Design review of the part built by this model. Coordinates are the model's own, in mm. A direction names the side the tool comes from. Round coordinates to 2 decimals unless told otherwise and drop trailing zeros. Order: outer loops, then holes, each group sorted by start corner. A loop starts at its lowest first (then second) coordinate and runs counter-clockwise, first axis right, second up. Notation, with made-up numbers: M 9.25,44 L 28.25,44 A15 cw 28.25,66 Z; hole C 43.25,7 d11. An arc over 180 degrees is marked long. Write each question's results on one line, items separated by ' | '. Start each with the question number.
Item 1: Take a section at B-B, the plane x = 95. Write out the cut boundary in (y, z).
Item 2: The part is to be moulded in two halves that separate along X. For faces 3 (the cylindrical face through (-112.4, 3.2, 91.7)), 4 (the flat face through (139.7, 3, 1)), 5 (the cylindrical face through (-136.08, 3.22, 110.48)), say which applies: +X half, -X half, draft (parallel to the pull), parting line (faces both ways), or undercut.
Item 3: Machinability: for faces 1 (the flat face through (114.3, 3, 1)), 2 (the flat face through (-2, 6.35, 100)), which of the approach directions +Z, -Z, +X, -X, +Y, -Y give a long, thin tool a straight path to every point of the face, cutting with its end or side? Answer none if there is none.
Item 4: Take a section at C-C, the plane y = 2.25. Count the separate pieces of the cut face and the enclosed holes in it, plus the area to 3 significant figures.
Item 5: Clearance check with flat-ended pins moving along their axes: pin 1 (3 mm diameter, centred on x = 69.85, z = 103.91, fed in from +Y); pin 2 (5 mm diameter, centred on x = 127, z = 57.15, fed in from -Y). State where each tip first meets the part, or that it passes through.
Item 6: Take a section at A-A, the plane z = 13.5. Write out the cut boundary in (x, y).
Item 7: Wall thickness on line 1 (X direction, y = 2, z = -57.15); line 2 (Z direction, x = -127, y = 2); line 3 (X direction, y = 2.5, z = -62): over which ranges is each line inside the solid? List them lowest first. Write a range as [from, to].
```python
from build123d import *

# Parameters (mm, degrees)
SKETCH1_W           = 279.4
SKETCH1_H           = 228.6
SKETCH1_W_2         = 228.6
SKETCH1_H_2         = 187.036363636
BOSS_EXTRUDE1_DEPTH = 6.35
SKETCH2_R           = 1.5875
CUT_EXTRUDE1_DEPTH  = 7.35
FILLET1_R           = 12.7
FILLET2_R           = 6.35


with BuildPart() as part:
    # Sketch1 → Boss-Extrude1 (new body)
    with BuildSketch(Plane(origin=(0, 0, 0), x_dir=(1, 0, 0), z_dir=(0, 1, 0))):
        Rectangle(SKETCH1_W, SKETCH1_H)
        Rectangle(SKETCH1_W_2, SKETCH1_H_2, mode=Mode.SUBTRACT)
    extrude(amount=BOSS_EXTRUDE1_DEPTH)

    # Sketch2 → Cut-Extrude1 (cut, through all)
    with BuildSketch(Plane(origin=(0, 6.35, 0), x_dir=(1, 0, 0), z_dir=(0, 1, 0))):
        with Locations((-63.5, 103.909090909)):
            Circle(SKETCH2_R)
        with Locations((-63.5, -103.909090909)):
            Circle(SKETCH2_R)
        with Locations((69.85, 103.909090909)):
            Circle(SKETCH2_R)
        with Locations((69.85, -103.909090909)):
            Circle(SKETCH2_R)
        with Locations((-127, 57.15)):
            Circle(SKETCH2_R)
        with Locations((-127, -57.15)):
            Circle(SKETCH2_R)
        with Locations((127, 57.15)):
            Circle(SKETCH2_R)
        with Locations((127, -57.15)):
            Circle(SKETCH2_R)
    extrude(amount=-CUT_EXTRUDE1_DEPTH, mode=Mode.SUBTRACT)

    # Fillet1
    fillet1_edges = [part.edges().sort_by_distance(p)[0] for p in [
        (139.7, 3.175, 114.3),
        (-139.7, 3.175, 114.3),
        (-139.7, 3.175, -114.3),
        (139.7, 3.175, -114.3),
    ]]
    fillet(fillet1_edges, radius=FILLET1_R)

    # Fillet2
    fillet2_edges = [part.edges().sort_by_distance(p)[0] for p in [
        (114.3, 3.175, 93.518181818),
        (114.3, 3.175, -93.518181818),
        (-114.3, 3.175, -93.518181818),
        (-114.3, 3.175, 93.518181818),
    ]]
    fillet(fillet2_edges, radius=FILLET2_R)


solid = part.part
```
Results list:
1) outline: M 0,-114.3 L 6.35,-114.3 L 6.35,-93.52 L 0,-93.52 Z; M 0,93.52 L 6.35,93.52 L 6.35,114.3 L 0,114.3 Z
2) face 3: undercut | face 4: +X half | face 5: -X half
3) face 1: +Y, -Y | face 2: +Z, -Z, +X, -X, +Y
4) separate pieces: 1 | enclosed holes: 9 | area: 20,900 mm²
5) pin 1: through | pin 2: y = 0
6) outline: M -139.7,0 L -114.3,0 L -114.3,6.35 L -139.7,6.35 Z; M 114.3,0 L 139.7,0 L 139.7,6.35 L 114.3,6.35 Z
7) line 1: [-139.7, -128.59], [-125.41, -114.3], [114.3, 125.41], [128.59, 139.7] | line 2: [-114.3, -58.74], [-55.56, 55.56], [58.74, 114.3] | line 3: [-139.7, -114.3], [114.3, 139.7]
